Input: part model. Units: mm. Frame: model coordinates. Round coordinates to 2 decimals unless told otherwise and drop trailing zeros. Loops run counter-clockwise (first coordinate to the right, second up) from the corner with the lowest first, then second, coordinate; pieces in that order, holes last. Notation, with made-up numbers: (-13.75, -25) - (1.25, -25) arc R14 ccw to (1.25, -1) - close; hole circle Ø10 at (63.25, 13). An arc over 180 degrees is marked (long way). One line per question, with ' | ' between items. Start each with the question number.
from build123d import *

# Parameters (mm, degrees)
F1_DEPTH = 450
F2_R     = 2.25
F3_DEPTH = 14.5
F4_R     = 4
F5_DEPTH = 6.2


with BuildPart() as f1:
    # F0 (on Front) → F1 (new body)
    with BuildSketch(Plane.XZ):
        with BuildLine():
            Line((-21, -7), (0, -7))
            Line((0, -7), (21, -7))
            Line((21, -7), (21, -3.8))
            ThreePointArc((21, -3.8), (20.292893, -3.507107), (20, -2.8))
            Line((20, -2.8), (18.2, -2.8))
            Line((18.2, -2.8), (18.2, -0.8))
            Line((18.2, -0.8), (20, -0.8))
            ThreePointArc((20, -0.8), (20.292893, -0.092893), (21, 0.2))
            Line((21, 0.2), (21, 6.792893))
            Line((21, 6.792893), (20.292893, 7.5))
            Line((20.292893, 7.5), (6, 7.5))
            Line((6, 7.5), (5.5, 7))
            Line((5.5, 7), (0, 7))
            Line((0, 7), (-5.5, 7))
            Line((-5.5, 7), (-6, 7.5))
            Line((-6, 7.5), (-20.292893, 7.5))
            Line((-20.292893, 7.5), (-21, 6.792893))
            Line((-21, 6.792893), (-21, 0.2))
            ThreePointArc((-21, 0.2), (-20.292893, -0.092893), (-20, -0.8))
            Line((-20, -0.8), (-18.2, -0.8))
            Line((-18.2, -0.8), (-18.2, -2.8))
            Line((-18.2, -2.8), (-20, -2.8))
            ThreePointArc((-20, -2.8), (-20.292893, -3.507107), (-21, -3.8))
            Line((-21, -3.8), (-21, -7))
        make_face()
    extrude(amount=-F1_DEPTH)

    # F2 (on face) → F3 (cut, through all)
    with BuildSketch(Plane.XY.offset(7.5)):
        with Locations((-12, 15)):
            Circle(F2_R)
        with Locations((-12, 75)):
            Circle(F2_R)
        with Locations((-12, 135)):
            Circle(F2_R)
        with Locations((-12, 375)):
            Circle(F2_R)
        with Locations((-12, 195)):
            Circle(F2_R)
        with Locations((-12, 255)):
            Circle(F2_R)
        with Locations((-12, 315)):
            Circle(F2_R)
        with Locations((-12, 435)):
            Circle(F2_R)
        with Locations((12, 15)):
            Circle(F2_R)
        with Locations((12, 435)):
            Circle(F2_R)
        with Locations((12, 315)):
            Circle(F2_R)
        with Locations((12, 75)):
            Circle(F2_R)
        with Locations((12, 135)):
            Circle(F2_R)
        with Locations((12, 195)):
            Circle(F2_R)
        with Locations((12, 255)):
            Circle(F2_R)
        with Locations((12, 375)):
            Circle(F2_R)
    extrude(amount=-F3_DEPTH, mode=Mode.SUBTRACT)

    # F4 (on face) → F5 (cut)
    with BuildSketch(Plane(origin=(0, 0, -7), x_dir=(1, 0, 0), z_dir=(0, 0, -1))):
        with Locations((-12, -435)):
            Circle(F4_R)
        with Locations((12, -435)):
            Circle(F4_R)
        with Locations((-12, -375)):
            Circle(F4_R)
        with Locations((12, -375)):
            Circle(F4_R)
        with Locations((-12, -315)):
            Circle(F4_R)
        with Locations((12, -315)):
            Circle(F4_R)
        with Locations((12, -255)):
            Circle(F4_R)
        with Locations((-12, -255)):
            Circle(F4_R)
        with Locations((-12, -195)):
            Circle(F4_R)
        with Locations((12, -195)):
            Circle(F4_R)
        with Locations((12, -135)):
            Circle(F4_R)
        with Locations((-12, -75)):
            Circle(F4_R)
        with Locations((-12, -135)):
            Circle(F4_R)
        with Locations((12, -75)):
            Circle(F4_R)
        with Locations((-12, -15)):
            Circle(F4_R)
        with Locations((12, -15)):
            Circle(F4_R)
    extrude(amount=-F5_DEPTH, mode=Mode.SUBTRACT)


solid = f1.part
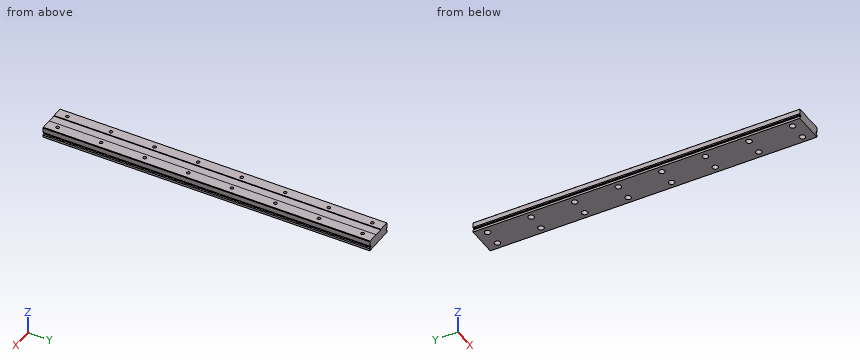
(1) Line query: line 1 along X through (y, z) = (435, -2.75); line 2 along X through (y, z) = (435, -3.5); line 3 along X through (y, z) = (124.5, -2). Output: solid intervals per line, ascending. Write a range as from..to.
(2) Section A-A, the plane y = 47.5. Output: boundary loops of the cut face in (x, z).
(3) Pin query (flat end, axial travel): P1, Ø5, axis at x = 12, y = 435, coming from the -Z side; P2, Ø5, axis at x = -12, y = 435, coming from the +Z side; P3, Ø2.5, axis at x = 12, y = 15, coming from the +Z side. Return the tip coordinate at first contact, or that it passes through.
Derived:
1) line 1: x = -18.2..-16, -8..8, 16..18.2 | line 2: x = -20.29..-16, -8..8, 16..20.29 | line 3: x = -18.2..18.2
2) outline: (-21, -7) - (21, -7) - (21, -3.8) arc R1 cw to (20, -2.8) - (18.2, -2.8) - (18.2, -0.8) - (20, -0.8) arc R1 cw to (21, 0.2) - (21, 6.79) - (20.29, 7.5) - (6, 7.5) - (5.5, 7) - (-5.5, 7) - (-6, 7.5) - (-20.29, 7.5) - (-21, 6.79) - (-21, 0.2) arc R1 cw to (-20, -0.8) - (-18.2, -0.8) - (-18.2, -2.8) - (-20, -2.8) arc R1 cw to (-21, -3.8) - close
3) P1: stops at z = -0.8 | P2: stops at z = 7.5 | P3: passes through
